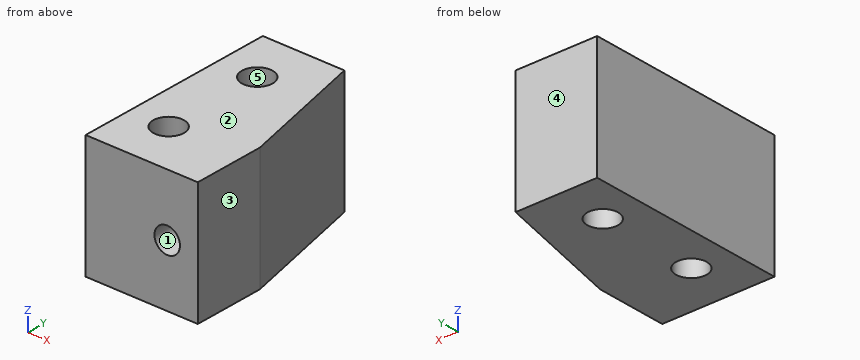
```python
from build123d import *

# Parameters (mm, degrees)
SKETCH_1_W               = 8
SKETCH_1_H               = 20
SKETCH_1_R               = 1.5
EXTRUDE_1_DEPTH          = 12
EXTRUDE_2_DEPTH          = 12
CUT_EXTRUDE_1_DEPTH      = 26.787593916
CUT_EXTRUDE_1_DEPTH_BACK = 7
SKETCH_3_R               = 1.25


with BuildPart() as part:
    # 草图1 → 凸台-拉伸1 (new body)
    with BuildSketch(Plane.XY):
        with Locations((4, 10)):
            Rectangle(SKETCH_1_W, SKETCH_1_H)
        with Locations((3.8, 15)):
            Circle(SKETCH_1_R, mode=Mode.SUBTRACT)
        with Locations(Location((3.8, 5, 0), (0, 0, 180))):
            Circle(SKETCH_1_R, mode=Mode.SUBTRACT)
    extrude(amount=EXTRUDE_1_DEPTH)

    # 草图2 → 凸台-拉伸2 (add)
    with BuildSketch(Plane.XY.offset(12)):
        Polygon((8, 20), (11, 7), (11, 0), (8, 0), align=None)
    extrude(amount=-EXTRUDE_2_DEPTH)

    # 草图3 → 切除-拉伸1 (cut, two sides: drawn at the far end of the back side and taken through both)
    with BuildSketch(Plane.XZ.offset(-CUT_EXTRUDE_1_DEPTH_BACK)):
        with Locations(Location((8, 6, 0), (0, 0, 90))):
            Circle(SKETCH_3_R)
    extrude(amount=CUT_EXTRUDE_1_DEPTH + CUT_EXTRUDE_1_DEPTH_BACK, mode=Mode.SUBTRACT)


solid = part.part
```
CAD build for the part. Positions are in the model's coordinates, mm. Face numbers are marked on the shaded views. A direction names the side the tool comes from. Round coordinates to 2 decimals unless told otherwise and drop trailing zeros. Order: outer loops, then holes, each group sorted by start corner. A loop starts at its lowest first (then second) coordinate and runs counter-clockwise, first axis right, second up.
Q1. Two-plate mould, pull along Y, no slides. Class the marked faces 3, 4 and 5: pulls with the +Y half, pulls with the -Y half, needs draft (parallel to the pull), parting line crosses it, or undercut.
Q2. Slice it at B-B (x = 3.8). Write the cut outline in (y, z), and give its area (3 significant figures).
Q3. Slice it at C-C (z = 4.5). Write the cut outline in (x, y), and give its area (3 significant figures).
Q4. Wall check: L1, parallel to Y at x = 3.8, z = 9.25; L2, parallel to Y at x = 4.5, z = 3; L3, parallel to X at y = 2.5, z = 6. Give the ranges that are in metal, low to high.
Q5. Slice it at A-A (y = 5). Write the cut outline in (x, z).
Q6. Slice it at D-D (y = 14.25). Write the cut outline in (x, z).
Q7. Drop flat-ended pins along their axis: pin 1 (1 mm diameter, centred on y = 11.5, z = 3.5, fed in from +X); pin 2 (0.8 mm diameter, centred on x = 7.5, z = 5.5, fed in from -Y). Give the stop position or say it passes through.
Q8. Which spindle directions (+Z, -Z, +X, -X, +Y, -Y) get a long thin tool onto all of the face, cutting with end or side? Do the marked faces 1 and 2. Say none if no direction does.
Results below:
1. face 3: needs draft
1. face 4: pulls with the +Y half
1. face 5: undercut
2. outline: (0, 0) - (3.5, 0) - (3.5, 12) - (0, 12) - close; (6.5, 0) - (13.5, 0) - (13.5, 12) - (6.5, 12) - close; (16.5, 0) - (20, 0) - (20, 12) - (16.5, 12) - close
2. area: 168 mm2
3. outline: (0, 0) - (11, 0) - (11, 7) - (8, 20) - (0, 20) - close; hole circle Ø3 at (3.8, 5); hole circle Ø3 at (3.8, 15)
3. area: 186 mm2
4. L1: y = 0 to 3.5, 6.5 to 13.5, 16.5 to 20
4. L2: y = 0 to 3.67, 6.33 to 13.67, 16.33 to 20
4. L3: x = 0 to 6.75, 9.25 to 11
5. outline: (0, 0) - (2.3, 0) - (2.3, 12) - (0, 12) - close; (5.3, 0) - (11, 0) - (11, 12) - (5.3, 12) - close; hole circle Ø2.5 at (8, 6)
6. outline: (0, 0) - (2.5, 0) - (2.5, 12) - (0, 12) - close; (5.1, 0) - (9.33, 0) - (9.33, 12) - (5.1, 12) - close
7. pin 1: stops at x = 10.08
7. pin 2: stops at y = 7
8. face 1: -Y
8. face 2: +Z, +X, -X, +Y, -Y
